from build123d import *

# Parameters (mm, degrees)
F1_DEPTH = 3.175


# Not quite as in the source:
# - a length typed as a fraction of an inch, garbled in the dataset ("3 / 203.2 mm" for 3/8 in), is restored


with BuildPart() as f1:
    # F0 (on Front) → F1 (new body)
    with BuildSketch(Plane.XZ):
        with BuildLine():
            Line((18.25, 0), (25.7, 0))
            ThreePointArc((25.7, 0), (23.7646270747, 9.7842986463), (18.25, 18.0949578612))
            Line((18.25, 18.0949578612), (18.25, 0))
        make_face()
        with BuildLine():
            ThreePointArc((-18.25, 18.0949578612), (-23.7646270747, 9.7842986463), (-25.7, 0))
            Line((-25.7, 0), (-18.25, 0))
            Line((-18.25, 0), (-18.25, 18.0949578612))
        make_face()
        with BuildLine():
            Line((14.75, 0), (14.75, 21.0458428199))
            ThreePointArc((14.75, 21.0458428199), (8.5638701474, 24.231180906), (1.75, 25.6403490616))
            Line((1.75, 25.6403490616), (1.75, 12.8201745308))
            Line((1.75, 12.8201745308), (1.75, 0))
            Line((1.75, 0), (14.75, 0))
        make_face()
        with BuildLine():
            Line((-14.75, 0), (-1.75, 0))
            Line((-1.75, 0), (-1.75, 12.8201745308))
            Line((-1.75, 12.8201745308), (-1.75, 25.6403490616))
            ThreePointArc((-1.75, 25.6403490616), (-8.5638701474, 24.231180906), (-14.75, 21.0458428199))
            Line((-14.75, 21.0458428199), (-14.75, 0))
        make_face()
        with BuildLine():
            ThreePointArc((-25.7, 0), (-18.1726442765, -18.1726442765), (0, -25.7))
            Line((0, -25.7), (0, 0))
            Line((0, 0), (-1.75, 0))
            Line((-1.75, 0), (-14.75, 0))
            Line((-14.75, 0), (-18.25, 0))
            Line((-18.25, 0), (-25.7, 0))
        make_face()
        with BuildLine():
            ThreePointArc((0, -25.7), (18.1726442765, -18.1726442765), (25.7, 0))
            Line((25.7, 0), (18.25, 0))
            Line((18.25, 0), (14.75, 0))
            Line((14.75, 0), (1.75, 0))
            Line((1.75, 0), (0, 0))
            Line((0, 0), (0, -25.7))
        make_face()
    extrude(amount=F1_DEPTH)


solid = f1.part
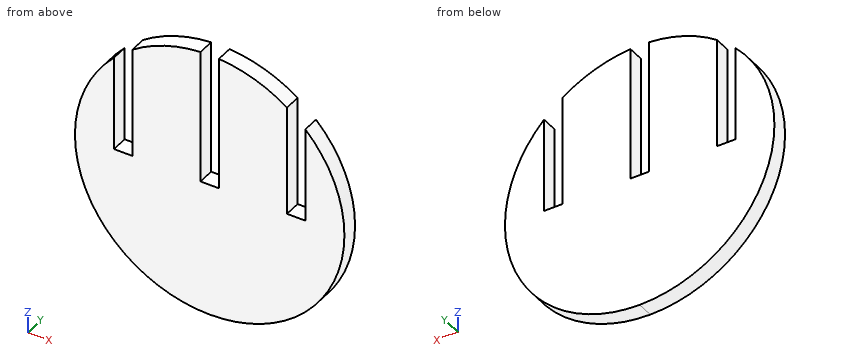
CAD build for the part. Positions are in the model's coordinates, mm. Give positions to 0.01 mm unless a question says otherwise; leave off trailing zeros. Order: outer loops, then holes, each group sorted by start corner. A loop starts at its lowest first (then second) coordinate and runs counter-clockwise, first axis right, second up. Notation, with made-up numbers: (54.25, 53.5) - (99.25, 53.5) arc R21 ccw to (99.25, 78.5) - close; hole circle Ø8 at (63, 0). An arc over 180 degrees is marked (long way). Answer in a Markdown table with one row per item.
1. Flat gauge pins, fed straight in: pin 1 (1.5 mm diameter, centred on y = -1.5, z = 3, fed in from +X); pin 2 (1.6 mm diameter, centred on x = 17, y = -1.5, fed in from +Z); pin 3 (1 mm diameter, centred on y = -1, z = 8.5, fed in from +X). Where does each tip first touch, or does it go through?
Data:
| item | result |
|---|---|
| pin 1 | stops at x = 25.6 |
| pin 2 | stops at z = 0 |
| pin 3 | stops at x = 24.42 |
2. Saw through at B-B, the plane y = -1.7. Give the cut face in (x, z).
Data:
| item | result |
|---|---|
| outline | (-18.25, 0) - (-18.25, 18.09) arc R25.7 ccw (long way) to (18.25, 18.09) - (18.25, 0) - (14.75, 0) - (14.75, 21.05) arc R25.7 ccw to (1.75, 25.64) - (1.75, 0) - (-1.75, 0) - (-1.75, 25.64) arc R25.7 ccw to (-14.75, 21.05) - (-14.75, 0) - close |
3. Saw through at D-D, the plane z = -4.5. Give the cut face in (x, y) (3 decimals), plus the area to 3 significant figures.
Data:
| item | result |
|---|---|
| outline | (-25.303, -3.175) - (25.303, -3.175) - (25.303, 0) - (-25.303, 0) - close |
| area | 161 mm² |
4. Saw through at A-A, the plane z = 17. Give the cut face in (x, y) (3 decimals), plus the area to 3 significant figures.
Data:
| item | result |
|---|---|
| outline | (-19.274, -3.175) - (-18.25, -3.175) - (-18.25, 0) - (-19.274, 0) - close; (-14.75, -3.175) - (-1.75, -3.175) - (-1.75, 0) - (-14.75, 0) - close; (1.75, -3.175) - (14.75, -3.175) - (14.75, 0) - (1.75, 0) - close; (18.25, -3.175) - (19.274, -3.175) - (19.274, 0) - (18.25, 0) - close |
| area | 89.1 mm² |
5. Probe probe 1 along X at (y, z) = (-0.7, 18.5); probe 2 along X at (y, z) = (-1.3, 11); probe 3 along X at (y, z) = (-2.65, 3). List the from-to ranges inside material, lowest first. Write a range as [from, to].
Data:
| item | result |
|---|---|
| probe 1 | x = [-14.75, -1.75], [1.75, 14.75] |
| probe 2 | x = [-23.23, -18.25], [-14.75, -1.75], [1.75, 14.75], [18.25, 23.23] |
| probe 3 | x = [-25.52, -18.25], [-14.75, -1.75], [1.75, 14.75], [18.25, 25.52] |
6. Saw through at C-C, the plane x = 1. Give the cut face in (y, z) (3 decimals).
Data:
| item | result |
|---|---|
| outline | (-3.175, -25.681) - (0, -25.681) - (0, 0) - (-3.175, 0) - close |
